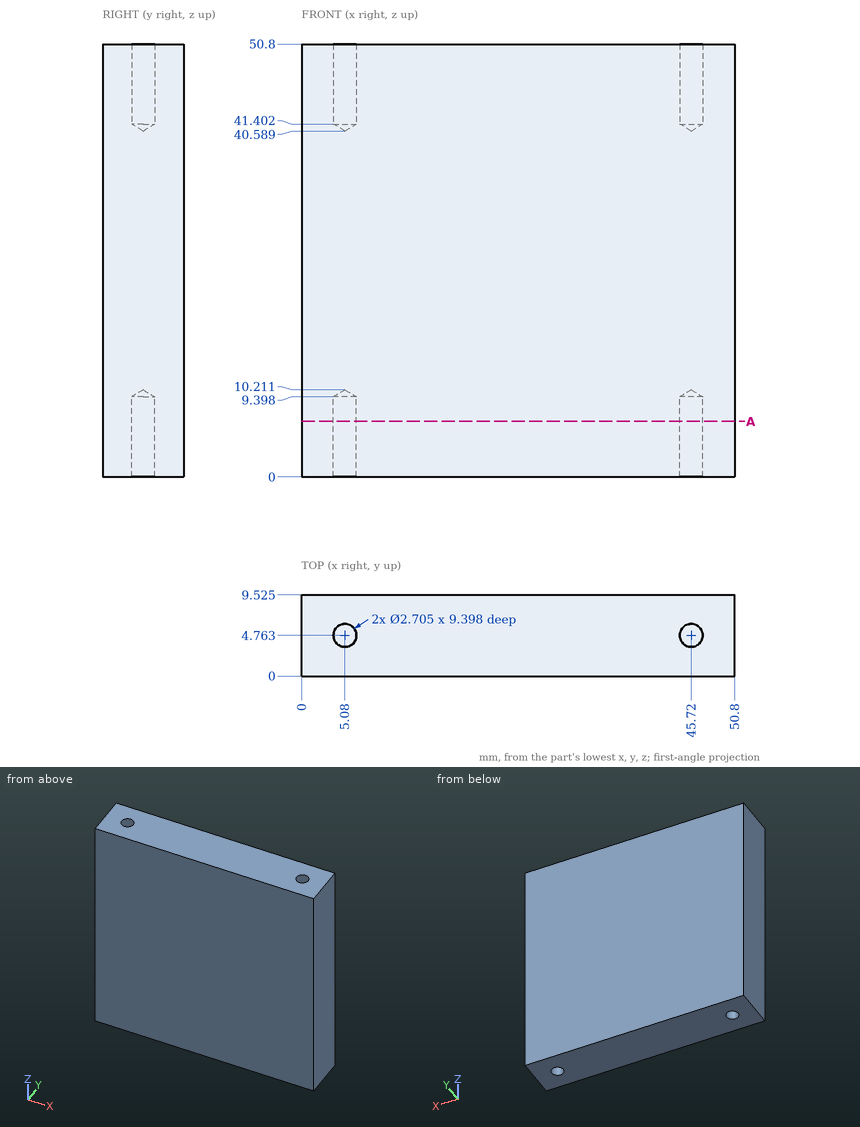
Geometry: see drawing. Coordinates: mm, zero at the bounding-box minimum. Coordinates: 2 decimals unless noted, no trailing zeros. Loops run counter-clockwise (first coordinate to the right, second up) from the corner with the lowest first, then second, coordinate; pieces in that order, holes last. Notation, with made-up numbers: (-34.5, 76.5) - (-4.5, 76.5) arc R8 cw to (-4.5, 84.5) - close; hole circle Ø10 at (79, 75.25). An arc over 180 degrees is marked (long way). Put each result on its own line as item: value. Start each with the question number.
Q1. Cut plane A-A, the plane z = 6.5. Return loops of the section in (x, y) (1 decimal).
Q2. Pin query (flat end, axial travel): pin 1 Ø1.6 at (x, y) = (5.08, 4.76) entering from +Z; pin 2 Ø2 at (x, y) = (5.08, 4.76) entering from -Z. Return the tip coordinate at first contact, or that it passes through.
Q3. Line query: line 1 (Y direction, x = 45.72, z = 44.25) (1 decimal); line 2 (X direction, y = 5.25, z = 46.5); line 3 (X direction, y = 5.75, z = 45) (1 decimal). Output: solid intervals per line, ascending.
Filled sheet:
1. outline: (0, 0) - (50.8, 0) - (50.8, 9.5) - (0, 9.5) - close; hole circle Ø2.7 at (5.1, 4.8); hole circle Ø2.7 at (45.7, 4.8)
2. pin 1: z = 41.07
2. pin 2: z = 9.61
3. line 1: 0 to 3.4, 6.1 to 9.5
3. line 2: 0 to 3.82, 6.34 to 44.46, 46.98 to 50.8
3. line 3: 0 to 4.2, 6 to 44.8, 46.6 to 50.8
